from build123d import *

# Parameters (mm, degrees)
SKETCH1_W           = 38.1
SKETCH1_H           = 38.1
SKETCH1_R           = 1.016
BOSS_EXTRUDE1_DEPTH = 2.54
FILLET1_R           = 6.35
FILLET2_R           = 0.5


with BuildPart() as part:
    # Sketch1 → Boss-Extrude1 (new body)
    with BuildSketch(Plane(origin=(0, 0, 0), x_dir=(1, 0, 0), z_dir=(0, 1, 0))):
        Rectangle(SKETCH1_W, SKETCH1_H)
        with Locations(Location((-14.986, 14.986, 0), (0, 0, 270))):
            Circle(SKETCH1_R, mode=Mode.SUBTRACT)
        with Locations(Location((-14.986, -14.986, 0), (0, 0, 270))):
            Circle(SKETCH1_R, mode=Mode.SUBTRACT)
        with Locations(Location((14.986, -14.986, 0), (0, 0, 270))):
            Circle(SKETCH1_R, mode=Mode.SUBTRACT)
        with Locations(Location((14.986, 14.986, 0), (0, 0, 270))):
            Circle(SKETCH1_R, mode=Mode.SUBTRACT)
    extrude(amount=BOSS_EXTRUDE1_DEPTH)

    # Fillet1
    fillet1_edges = [part.edges().sort_by_distance(p)[0] for p in [
        (-19.05, 1.27, -19.05),
        (19.05, 1.27, -19.05),
        (19.05, 1.27, 19.05),
        (-19.05, 1.27, 19.05),
    ]]
    fillet(fillet1_edges, radius=FILLET1_R)

    # Fillet2
    fillet2_edges = [part.edges().sort_by_distance(p)[0] for p in [
        (-14.986, 0, -16.002),
        (-14.986, 0, 13.97),
        (14.986, 0, 13.97),
        (14.986, 0, -16.002),
    ]]
    fillet(fillet2_edges, radius=FILLET2_R)


solid = part.part
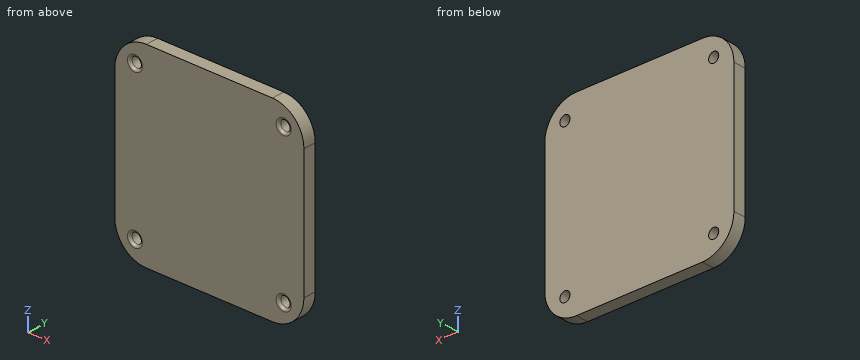
Read the model definition and answer for the solid it produces. Units are mm, in the model's axes. Round coordinates to 2 decimals unless told otherwise and drop trailing zeros. Order: outer loops, then holes, each group sorted by start corner. A loop starts at its lowest first (then second) coordinate and runs counter-clockwise, first axis right, second up. Notation, with made-up numbers: (-11.5, 26) - (-4.5, 26) arc R26 ccw to (-4.5, 52) - close; hole circle Ø9 at (24, 62). An arc over 180 degrees is marked (long way). Use one line per item in the form item = value. Start each with the question number.
(1) The part is cut by section A-A (y = 0.95). Give the vertices of the cut face in (x, z).
(2) A flat-ended cylindrical pin translates along its axis: pin 1 Ø2.5 at (x, z) = (14.986, -14.986) entering from -Y. Find the tip coordinate at first contact, or state that the pin passes through.
(3) Find the intervals of material crossed by line 1 along Z through (x, y) = (15, 0.25); line 2 along X through (y, z) = (0.45, 15.5); line 3 along X through (y, z) = (1.45, 15), in increasing order. Write a range as from..to.
Checked values:
q1.outline = (-19.05, -12.7) arc R6.35 ccw to (-12.7, -19.05) - (12.7, -19.05) arc R6.35 ccw to (19.05, -12.7) - (19.05, 12.7) arc R6.35 ccw to (12.7, 19.05) - (-12.7, 19.05) arc R6.35 ccw to (-19.05, 12.7) - close; hole circle Ø2.03 at (-14.99, -14.99); hole circle Ø2.03 at (-14.99, 14.99); hole circle Ø2.03 at (14.99, -14.99); hole circle Ø2.03 at (14.99, 14.99)
q2.pin_1 = 0.08
q3.line_1 = -18.62..-16.07, -13.9..13.9, 16.07..18.62
q3.line_2 = -18.4..-15.87, -14.11..14.11, 15.87..18.4
q3.line_3 = -18.62..-16, -13.97..13.97, 16..18.62
